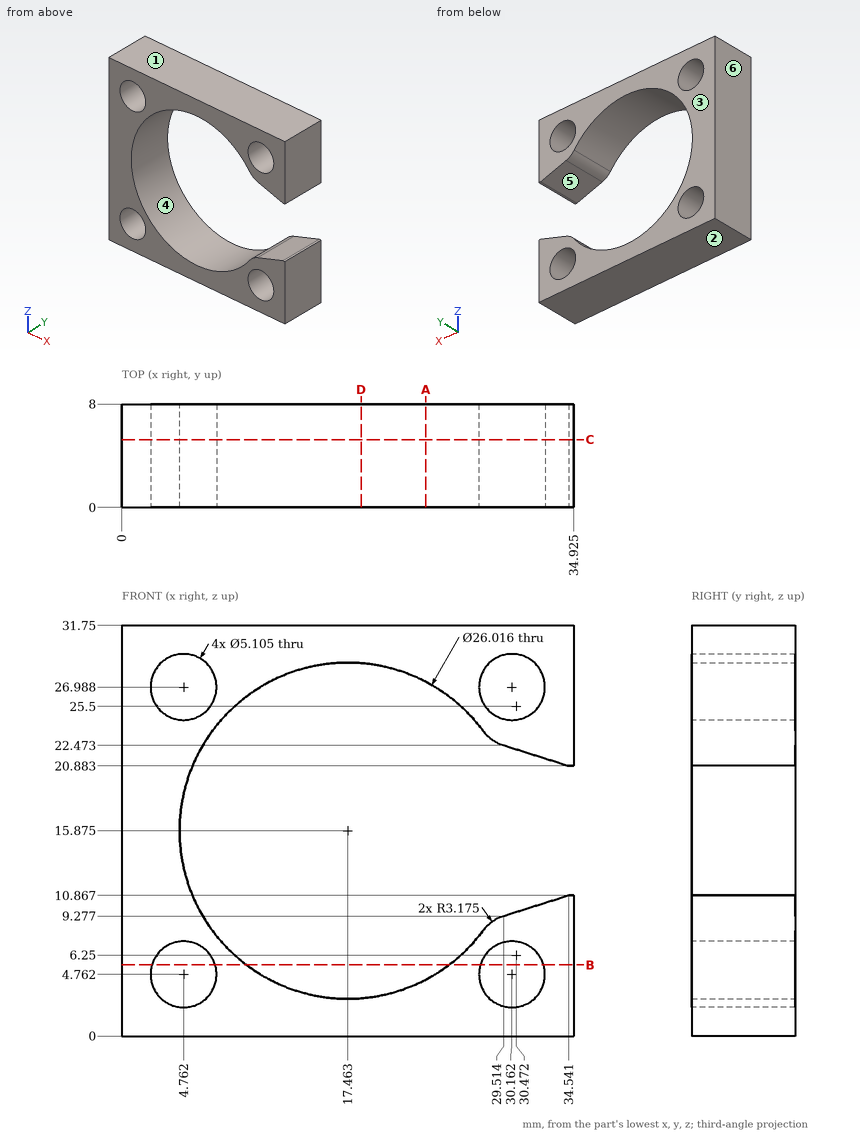
Design review of the part shown in the three views and the two pictorial views. Dimensions are in mm from the part's minimum x, y and z. A direction names the side the tool comes from. Give positions to 0.01 mm unless a question says otherwise; leave off trailing zeros. Order: outer loops, then holes, each group sorted by start corner. A loop starts at its lowest first (then second) coordinate and runs counter-clockwise, first axis right, second up. Notation, with made-up numbers: M 29.5,47.25 L 43.5,47.25 A26 cw 43.5,78.25 Z; hole C -10,-15.75 d10. An arc over 180 degrees is marked long. Answer in a Markdown table with one row per item. Add a question column.
(1) Consider section D-D on x = 18.5. State the section outline as (y, z) points.
(2) Consider section A-A on x = 23.5. State the section outline as (y, z) points.
(3) Wall thickness on probe 1 along X at (y, z) = (5, 25) (1 decimal); probe 2 along Z at (x, y) = (17.5, 2.25); probe 3 along X at (y, z) = (7.5, 27) (1 decimal): over which ranges is each line inside the solid? List them lowest first. Write a range as [from, to].
(4) Consider section C-C on y = 5.25. Give the number of separate pieces and of enclosed holes in the cut face.
(5) Consider section B-B on z = 5.5. State the section outline as (x, y) points (1 decimal).
(6) For the marked faces 5 and 6, list the 3-axis set-ups (+Z, -Z, +X, -X, +Y, -Y) from which the entire face can be reached by the end or side of a thin tool; tool diameter is ignored.
(7) For pin 1 (1 mm diameter, centred on y = 5, z = 20, fed in from +X) (1 decimal), flat-tipped, find the tip position at first contact; note if it passes through.
(8) Mouldability with a two-part tool opening along Z and no side actions: class the marked faces 1, 2, 3 and 4 as +Z half, -Z half, draft (parallel to the pull), parting line (faces both ways), or undercut.
Evaluation:
| question | item | result |
|---|---|---|
| 1 | outline | M 0,0 L 8,0 L 8,2.91 L 0,2.91 Z; M 0,28.84 L 8,28.84 L 8,31.75 L 0,31.75 Z |
| 2 | outline | M 0,0 L 8,0 L 8,4.35 L 0,4.35 Z; M 0,27.4 L 8,27.4 L 8,31.75 L 0,31.75 Z |
| 3 | probe 1 | x = [0, 3.2], [6.4, 8.2], [26.7, 28.6], [31.8, 34.9] |
| 3 | probe 2 | z = [0, 2.87], [28.88, 31.75] |
| 3 | probe 3 | x = [0, 2.2], [7.3, 10.7], [24.2, 27.6], [32.7, 34.9] |
| 4 | separate pieces | 1 |
| 4 | enclosed holes | 4 |
| 5 | outline | M 0,0 L 2.3,0 L 2.3,8 L 0,8 Z; M 7.2,0 L 9.6,0 L 9.6,8 L 7.2,8 Z; M 25.3,0 L 27.7,0 L 27.7,8 L 25.3,8 Z; M 32.6,0 L 34.9,0 L 34.9,8 L 32.6,8 Z |
| 6 | face 5 | +Y, -Y |
| 6 | face 6 | +Z, -Z, -X, +Y, -Y |
| 7 | pin 1 | stops at x = 5.3 |
| 8 | face 1 | +Z half |
| 8 | face 2 | -Z half |
| 8 | face 3 | draft |
| 8 | face 4 | undercut |
